Model file for the job. Use its own axes, mm. A direction names the side the tool comes from. Coordinates: 2 decimals unless noted, no trailing zeros. Loops run counter-clockwise (first coordinate to the right, second up) from the corner with the lowest first, then second, coordinate; pieces in that order, holes last. Notation, with made-up numbers: (25.5, -24.75) -> (82.5, -24.75) arc R9 ccw to (82.5, -18.75) -> close; hole circle Ø11 at (10, 17.25). An arc over 180 degrees is marked (long way). Use one line per item in the form item = value.
Autodesk Inventor part; units mm, degrees
ref_plane "YZ Plane" through (0, 0, 0) normal (1, 0, 0) x (0, 1, 0)
ref_plane "XZ Plane" through (0, 0, 0) normal (0, 1, 0) x (-1, 0, 0)
ref_plane "XY Plane" through (0, 0, 0) normal (0, 0, 1) x (1, 0, 0)
sketch "Sketch1" plane through (0, 0, 0) normal (0, 0, 1) x (1, 0, 0)
  line L0 (0, 27.432) -> (-109.1184, 73.152)
  line L1 (-109.1184, 73.152) -> (-161.8488, 208.4832)
  line L2 (-161.8488, 208.4832) -> (0, 264.2616)
  line L3 (0, 562.8605) -> (0, -145.2705) construction
  line L4 (0, 264.2616) -> (0, 27.432)
  point P0 (0, 0)
  dimension "d9" = 264.2616
  dimension "d11" = 161.8488
  dimension "d15" = 208.4832
  dimension "d20" = 109.1184
  dimension "d22" = 73.152
  dimension "d39" = 0
  dimension "d41" = 0
  dimension "d42" = 27.432
extrude "Extrusion4" add sketch "Sketch1" along normal blind 18
hole "Hole2" at (0.0182, 257.4006, 18) direction (0, 0, -1) diameter 15 end through all
hole "Hole3" at (-155.3023, 205.1164, 18) direction (0, 0, -1) diameter 15 end through all
hole "Hole4" at (-104.3588, 77.9489, 18) direction (0, 0, -1) diameter 15 end through all
hole "Hole5" at (0.2097, 34.0914, 18) direction (0, 0, -1) diameter 15 end through all
fillet "Fillet7" radius 1.5 1 edges at (-5.647, 262.3155, 9)
fillet "Fillet8" radius 1 1 edges at (-152.0327, 211.8661, 9)
fillet "Fillet9" radius 1 1 edges at (-157.7785, 198.0369, 9)
fillet "Fillet10" radius 2 1 edges at (-111.6584, 79.6709, 9)
fillet "Fillet11" radius 2 1 edges at (-102.9745, 70.5777, 9)
fillet "Fillet12" radius 2 1 edges at (-6.056, 29.9694, 9)
sketch "Sketch5" plane through (0, 0, 18) normal (0, 0, 1) x (1, 0, 0)
  line L0 (0, 41.5885) -> (0, 249.9006)
  line L1 (-91.2304, 90.5943) -> (-131.73, 194.5356)
  line L2 (-131.73, 194.5356) -> (-30, 229.5951)
  line L3 (-30, 229.5951) -> (0, 229.5951)
  line L4 (-9.1769, 261.0989) -> (-150.1114, 212.5283)
  line L5 (-157.1008, 196.2976) -> (-113.2116, 83.657)
  line L6 (-98.9493, 68.8912) -> (-10.0438, 31.6403)
  line L7 (-91.2304, 90.5943) -> (-30, 64.9391)
  line L8 (-30, 64.9391) -> (0, 64.9391)
  point P0 (0, 0)
  dimension "d148" = 23
  dimension "d149" = 23
  dimension "d151" = 23
  dimension "d152" = 30
  dimension "d153" = 30
extrude "Extrusion5" cut sketch "Sketch5" against normal through all
fillet "Fillet14" radius 40 1 edges at (-131.73, 194.5356, 9)
fillet "Fillet15" radius 100 1 edges at (-30, 229.5951, 9)
fillet "Fillet16" radius 150 1 edges at (-91.2304, 90.5943, 9)
fillet "Fillet17" radius 50 1 edges at (-30, 64.9391, 9)
mirror "Mirror2" about plane through (0, 0, 0) normal (1, 0, 0)
properties part number "section1" material "Polyethylene, High Density"
Q1. Which spindle directions (+Z, -Z, +X, -X, +Y, -Y) get a long thin tool onto all of the face, cutting with end or side? Do faces 1 (the face through (11, 232, 0)), 2 (the face through (0, 229.595, 9)). Say none if no direction does.
Result:
face_1 = -Z, +X, -X, +Y, -Y
face_2 = +Z, -Z
Q2. Band-saw the part on A-A, the plane y = 93. Write the cut outline in (x, z), and give its area (3 significant figures).
Result:
outline = (-116.85, 0) -> (-75.08, 0) -> (-75.08, 18) -> (-116.85, 18) -> close; (75.08, 0) -> (116.85, 0) -> (116.85, 18) -> (75.08, 18) -> close
area = 1,500 mm2
Q3. Band-saw the part on B-B, the plane x = 83.5. Write the cut outline in (y, z), and give its area (3 significant figures).
Result:
outline = (62.42, 0) -> (101.23, 0) -> (101.23, 18) -> (62.42, 18) -> close; (211.16, 0) -> (235.48, 0) -> (235.48, 18) -> (211.16, 18) -> close
area = 1,140 mm2
Q4. Pin check, flat tips, straight feed: pin 1 Ø3 at (y, z) = (213.5, 14) entering from +X; pin 2 Ø8 at (x, z) = (-118, 8.5) entering from +Y; pin 3 Ø8 at (y, z) = (91.5, 3.5) entering from +X. Stop position of each tip, or through.
Result:
pin_1 = 150.69
pin_2 = 224.97
pin_3 = 117.83
Q5. Mould opens along Y. For faces 3 (the face through (-29.999, 228.183, 8.874)), 4 (the face through (78.658, 237.154, 8.874)), 5 (the face through (135.463, 140.766, 8.874)) say: released by +Y, released by -Y, zero draft, split by the parting line, or undercut.
Result:
face_3 = undercut
face_4 = released by +Y
face_5 = released by -Y
Q6. Wall check: line 1 along Y through (x, z) = (17, 13.75); line 2 along X through (y, z) = (153.5, 11.25); line 3 along X through (y, z) = (149.5, 8.25). Give the ranges that are in metal, low to high.
Result:
line_1 = 34.55 to 64.94, 229.52 to 258.4
line_2 = -140.43 to -115.74, 115.74 to 140.43
line_3 = -138.87 to -114.18, 114.18 to 138.87
Q7. Band-saw the part on D-D, the plane y = 245. Write the cut outline in (x, z).
Result:
outline = (-55.89, 0) -> (55.89, 0) -> (55.89, 18) -> (-55.89, 18) -> close
Q8. Band-saw the part on C-C, the plane y = 61. Write the cut outline in (x, z).
Result:
outline = (-80.12, 0) -> (80.12, 0) -> (80.12, 18) -> (-80.12, 18) -> close
